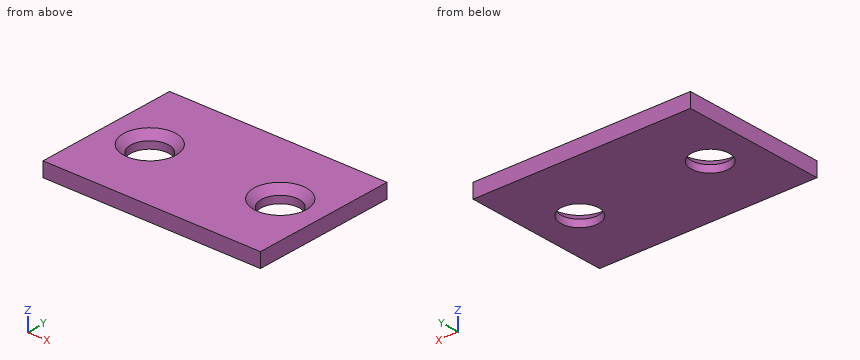
```python
from build123d import *

# Parameters (mm, degrees)
SKETCH1_W          = 30
SKETCH1_H          = 20
BASE_FLANGE1_DEPTH = 2


# Sheet-metal steps are written as plain solids
with BuildPart() as part:
    # Sketch1 → Base-Flange1 (new body)
    with BuildSketch(Plane.XY):
        Rectangle(SKETCH1_W, SKETCH1_H)
    extrude(amount=BASE_FLANGE1_DEPTH)

    # Sketch6 → Ø5.2 (5.2) Diameter Hole1 (revolve, cut)
    with BuildSketch(Plane(origin=(-9, 0, 2), x_dir=(0, -1, 0), z_dir=(1, 0, 0))):
        Polygon((0, 0), (0, 2), (2.6, 2), (2.6, 1), (3.6, 0), align=None)
    f_5_2_5_2_diameter_hole1 = revolve(axis=Axis((-9, 0, 8.35), (0, 0, -1)), mode=Mode.SUBTRACT)

    # Mirror1: Ø5.2 (5.2) Diameter Hole1 across plane
    add(f_5_2_5_2_diameter_hole1.mirror(Plane(origin=(0, 0, 0), x_dir=(0, 0, 1), z_dir=(1, 0, 0))), mode=Mode.SUBTRACT)


solid = part.part
```
Check sheet for the modelled part. Datum: model origin and axes. Units: mm. Round coordinates to 2 decimals unless told otherwise and drop trailing zeros. Order: outer loops, then holes, each group sorted by start corner. A loop starts at its lowest first (then second) coordinate and runs counter-clockwise, first axis right, second up. Notation, with made-up numbers: M -16.75,52.25 L 1.25,52.25 A19 ccw 1.25,72.25 Z; hole C 87.5,5.5 d4. An arc over 180 degrees is marked long. Answer in a Markdown table with one row per item.
(1) Section check C-C on z = 1.65. Record the boundary of the cut face in (x, y).
Findings:
| item | result |
|---|---|
| outline | M -15,-10 L 15,-10 L 15,10 L -15,10 Z; hole C -9,0 d6.5; hole C 9,0 d6.5 |
(2) Material ranges on line 1 along X through (y, z) = (0, 0.2); line 2 along X through (y, z) = (-0.5, 1.15); line 3 along Y through (x, z) = (-9, 0.25), recorded low to high. Write a range as from..to.
Findings:
| item | result |
|---|---|
| line 1 | x = -15..-11.6, -6.4..6.4, 11.6..15 |
| line 2 | x = -15..-11.7, -6.3..6.3, 11.7..15 |
| line 3 | y = -10..-2.6, 2.6..10 |
(3) Section check A-A on x = 9. Record the boundary of the cut face in (y, z), plus the area to 3 significant figures.
Findings:
| item | result |
|---|---|
| outline | M -10,0 L -2.6,0 L -2.6,1 L -3.6,2 L -10,2 Z; M 2.6,0 L 10,0 L 10,2 L 3.6,2 L 2.6,1 Z |
| area | 28.6 mm^2 |
(4) Section check B-B on y = 0. Record the boundary of the cut face in (x, z).
Findings:
| item | result |
|---|---|
| outline | M -15,0 L -11.6,0 L -11.6,1 L -12.6,2 L -15,2 Z; M -6.4,0 L 6.4,0 L 6.4,1 L 5.4,2 L -5.4,2 L -6.4,1 Z; M 11.6,0 L 15,0 L 15,2 L 12.6,2 L 11.6,1 Z |
